```python
from build123d import *

# Parameters (mm, degrees)
SKETCH1_R            = 2.1
BOSS_EXTRUDE2_DEPTH  = 422
CUT_EXTRUDE1_DEPTH   = 423.236900478
FILLET1_R            = 0.25
FILLET1_OF_MIRROR1_R = 0.25


with BuildPart() as part:
    # Sketch1 → Boss-Extrude2 (new body)
    with BuildSketch(Plane.XY):
        Polygon((8.199993721, -10), (9.999993721, -10), (9.999993721, -4.63999575), (8.199993721, -2.84), (8.199993721, -5.800653822), (6.861313026, -5.800653822), (3.900652213, -2.84), (3.900652213, 2.84), (6.559993721, 5.499347787), (8.199993721, 5.499347787), (8.199993721, 2.84), (9.999993721, 4.64000425), (9.999993721, 10), (4.63999575, 10), (2.84, 8.2), (5.499325592, 8.2), (5.499325592, 6.56), (2.84, 3.900668129), (-2.84, 3.900668129), (-5.49933815, 6.56), (-5.49933815, 8.2), (-2.84, 8.2), (-4.64000425, 10), (-10.000006279, 10), (-10.000006279, 4.63999575), (-8.200006279, 2.84), (-8.200006279, 5.499347787), (-6.560006279, 5.499347787), (-3.900652213, 2.84), (-3.900652213, -2.84), (-6.861299044, -5.800653822), (-8.200006279, -5.800653822), (-8.200006279, -2.84), (-10.000006279, -4.64000425), (-10.000006279, -10), (-8.200006279, -10), (-8.200006279, -7.300653822), (-6.239977665, -7.300653822), (-2.84, -3.900668129), (2.84, -3.900668129), (6.239993721, -7.300653822), (8.199993721, -7.300653822), align=None)
        with Locations(Location((0, 0, 0), (0, 0, 180))):
            Circle(SKETCH1_R, mode=Mode.SUBTRACT)
    boss_extrude2 = extrude(amount=BOSS_EXTRUDE2_DEPTH)

    # Sketch2 → Cut-Extrude1 (cut, through all)
    with BuildSketch(Plane.XY.offset(422)):
        Polygon((-8.200006279, 6.569347787), (-8.200006279, 8.2), (-6.56933815, 8.2), (-6.56933815, 7.630009211), (-7.62999707, 6.569347787), align=None)
        Polygon((8.199993721, 8.2), (8.199993721, 6.569347787), (7.629987016, 6.569347787), (6.569325592, 7.630006706), (6.569325592, 8.2), align=None)
    cut_extrude1 = extrude(amount=-CUT_EXTRUDE1_DEPTH, mode=Mode.SUBTRACT)

    # Fillet1
    fillet1_edges = [part.edges().sort_by_distance(p)[0] for p in [
        (9.999993721, -4.63999575, 211),
        (-10.000006279, -4.64000425, 211),
        (-8.200006279, -2.84, 211),
        (-8.200006279, 2.84, 211),
        (-10.000006279, 4.63999575, 211),
        (-10.000006279, 10, 211),
        (-4.64000425, 10, 211),
        (-2.84, 8.2, 211),
        (2.84, 8.2, 211),
        (4.63999575, 10, 211),
        (9.999993721, 10, 211),
        (9.999993721, 4.64000425, 211),
        (8.199993721, 2.84, 211),
        (8.199993721, -2.84, 211),
    ]]
    fillet(fillet1_edges, radius=FILLET1_R)

    # Mirror1: Boss-Extrude2 across plane
    add(boss_extrude2.mirror(Plane(origin=(0, -10, 0), x_dir=(0, 0, 1), z_dir=(0, -1, 0))))

    # Fillet1 of Mirror1
    fillet1_of_mirror1_edges = [part.edges().sort_by_distance(p)[0] for p in [
        (9.999993721, -15.36000425, 211),
        (-10.000006279, -15.35999575, 211),
        (-8.200006279, -17.16, 211),
        (-8.200006279, -22.84, 211),
        (-10.000006279, -24.63999575, 211),
        (-10.000006279, -30, 211),
        (-4.64000425, -30, 211),
        (-2.84, -28.2, 211),
        (2.84, -28.2, 211),
        (4.63999575, -30, 211),
        (9.999993721, -30, 211),
        (9.999993721, -24.64000425, 211),
        (8.199993721, -22.84, 211),
        (8.199993721, -17.16, 211),
    ]]
    fillet(fillet1_of_mirror1_edges, radius=FILLET1_OF_MIRROR1_R)

    # Mirror2: Cut-Extrude1 across plane
    add(cut_extrude1.mirror(Plane(origin=(0, -10, 0), x_dir=(0, 0, 1), z_dir=(0, -1, 0))), mode=Mode.SUBTRACT)


solid = part.part
```
Can you work these out from the model? Positions are in its coordinate system, mm. Round coordinates to 2 decimals unless told otherwise and drop trailing zeros. Write item = value, one per line. Start each with the question number.
(1) I need wall thicknesses on line 1 along Y through (x, z) = (0, 333); line 2 along Y through (x, z) = (8.75, 254); line 3 along X through (y, z) = (-15.5, 127.5). Which ranges of each line are inside material? Lowest first, please.
(2) Suppose I cut it at A-A on z = 198. Give the number of separate pieces and of enclosed holes in the cut face, plus the area to 3 significant figures.
(3) I'm going to push flat-ended pins straight in: P1, Ø2.5, axis at x = 0, y = -20, coming from the -Z side (3 decimals); P2, Ø12, axis at y = -19.5, z = 291, coming from the -X side; P3, Ø1.7, axis at y = -19.5, z = 160, coming from the -X side; P4, Ø3, axis at y = -22, z = 353.5, coming from the -X side. Where does each tip first touch, or does it pass through?
Answer block:
q1.line_1 = -23.9 to -22.1, -17.9 to -16.1, -3.9 to -2.1, 2.1 to 3.9
q1.line_2 = -30 to -23.39, -16.61 to -3.39, 3.39 to 10
q1.line_3 = -9.86 to -8.2, -5.56 to -3.44, 3.44 to 5.56, 8.2 to 9.86
q2.separate_pieces = 1
q2.enclosed_holes = 7
q2.area = 289 mm²
q3.P1 = through
q3.P2 = -10
q3.P3 = -3.9
q3.P4 = -8.86
